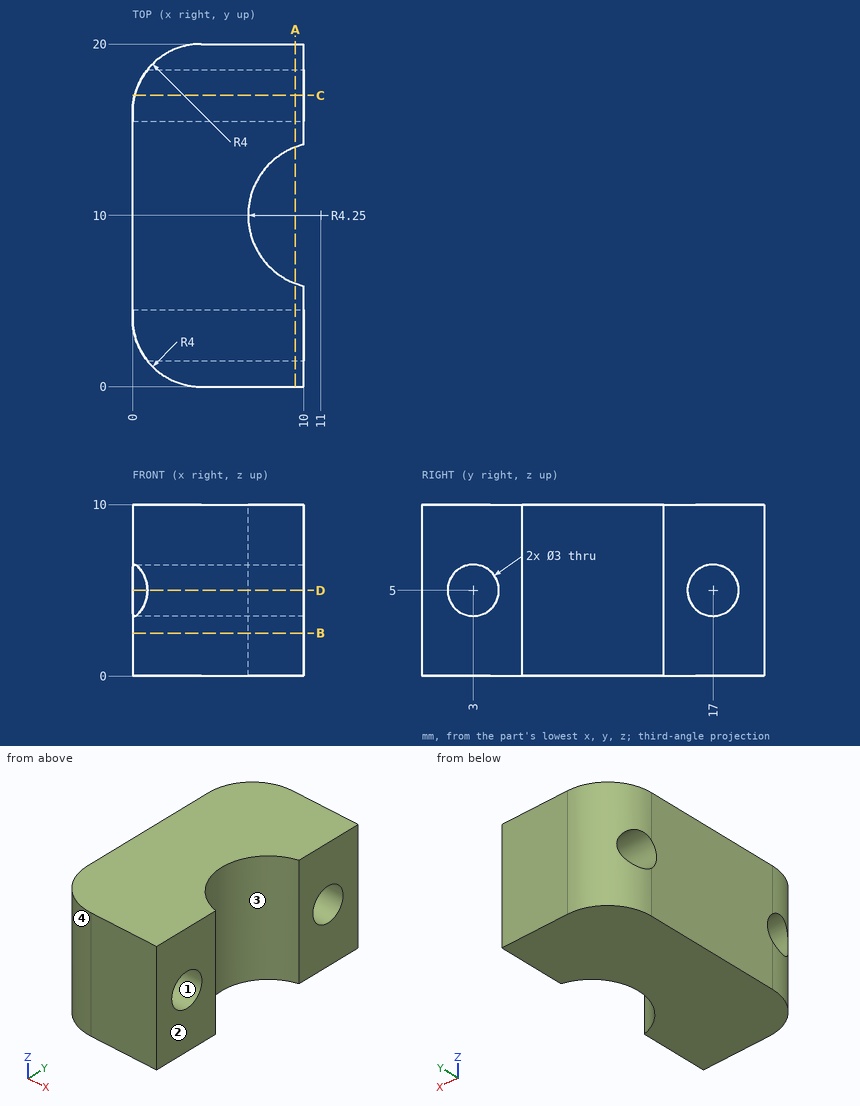
The drawing under review shows one solid part. Ordinate dimensions are in mm from its lowest x, y, z. Coordinates: 2 decimals unless noted, no trailing zeros. Order: outer loops, then holes, each group sorted by start corner. A loop starts at its lowest first (then second) coordinate and runs counter-clockwise, first axis right, second up. Notation, with made-up numbers: (44, -39) - (90, -39) arc R18 ccw to (90, -19) - close; hole circle Ø6 at (-8.75, 9). An arc over 180 degrees is marked (long way). Put each result on its own line as item: value.
1) Take a section at D-D, the plane z = 5. Give the boundary of the cut face in (x, y).
Response values:
outline: (0, 4.5) - (10, 4.5) - (10, 5.87) arc R4.25 cw to (10, 14.13) - (10, 15.5) - (0, 15.5) - close; (0.88, 1.5) arc R4 ccw to (4, 0) - (10, 0) - (10, 1.5) - close; (0.88, 18.5) - (10, 18.5) - (10, 20) - (4, 20) arc R4 ccw to start
2) Take a section at B-B, the plane z = 2.5. Give the boundary of the cut face in (x, y), and give its area (3 significant figures).
Response values:
outline: (0, 4) arc R4 ccw to (4, 0) - (10, 0) - (10, 5.87) arc R4.25 cw to (10, 14.13) - (10, 20) - (4, 20) arc R4 ccw to (0, 16) - close
area: 173 mm²
3) Wall thickness on L1, parallel to Y at x = 4.25, z = 5; L2, parallel to Y at x = 3.25, z = 5; L3, parallel to X at y = 10, z = 0.75: over which ranges is each line inside the solid? List them lowest first. Write a range as from..to.
Response values:
L1: y = 0..1.5, 4.5..15.5, 18.5..20
L2: y = 0.07..1.5, 4.5..15.5, 18.5..19.93
L3: x = 0..6.75
4) The part is to be moulded in two halves that separate along Y. For the marked faces 1, 2, 3 and 4, say which applies: released by +Y, released by -Y, zero draft, split by the parting line, or undercut.
Response values:
face 1: undercut
face 2: zero draft
face 3: undercut
face 4: released by -Y
5) Take a section at C-C, the plane y = 17. Give the boundary of the cut face in (x, z).
Response values:
outline: (0.13, 0) - (10, 0) - (10, 3.5) - (0.13, 3.5) - close; (0.13, 6.5) - (10, 6.5) - (10, 10) - (0.13, 10) - close
6) Take a section at A-A, the plane x = 9.5. Give the boundary of the cut face in (y, z).
Response values:
outline: (0, 0) - (6.02, 0) - (6.02, 10) - (0, 10) - close; (13.98, 0) - (20, 0) - (20, 10) - (13.98, 10) - close; hole circle Ø3 at (3, 5); hole circle Ø3 at (17, 5)
7) Insertion check: P1, Ø1.8, axis at y = 17, z = 5, coming from the +X side. The pin has a flat end and moves straight along its axis. Give the tip position at first contact, or say it passes through.
Response values:
P1: passes through
